Autodesk Inventor part; units mm, degrees
ref_plane "YZ Plane" through (0, 0, 0) normal (1, 0, 0) x (0, 1, 0)
ref_plane "XZ Plane" through (0, 0, 0) normal (0, 1, 0) x (-1, 0, 0)
ref_plane "XY Plane" through (0, 0, 0) normal (0, 0, 1) x (1, 0, 0)
sketch "スケッチ1" plane through (0, 0, 0) normal (1, 0, 0) x (0, 1, 0)
  line L0 (0, 0) -> (15, 0)
  line L1 (15, 0) -> (15, -150)
  line L2 (15, -150) -> (0, -150)
  line L3 (0, -150) -> (0, 0)
  line L4 (0, 0) -> (-40, 0)
  line L5 (-40, 0) -> (-40, -15)
  line L6 (-40, -15) -> (0, -15)
  line L7 (0, -15) -> (0, 0)
  line L8 (0, -150) -> (-40, -150)
  line L9 (-40, -150) -> (-40, -135)
  line L10 (-40, -135) -> (0, -135)
  line L11 (0, -135) -> (0, -150)
  dimension "d0" = 15
  dimension "d1" = 150
  dimension "d2" = 40
  dimension "d3" = 15
  dimension "d4" = 40
  dimension "d5" = 15
extrude "押し出し1" add sketch "スケッチ1" along normal blind 6
sketch "スケッチ2" plane through (6, 0, 0) normal (1, 0, 0) x (0, 0, -1)
  line L0 (150, 15) -> (0, 15)
  line L1 (0, 15) -> (0, -40)
  line L2 (75, 15) -> (75, -40) construction
  point P0 (0, 0)
  point P1 (7.5, 5)
  point P2 (7.5, -5)
  point P3 (7.5, -15)
  point P4 (25, 7.5)
  point P5 (35, 7.5)
  point P6 (45, 7.5)
  point P7 (142.5, 5)
  point P8 (142.5, -5)
  point P9 (142.5, -15)
  point P10 (125, 7.5)
  point P11 (115, 7.5)
  point P12 (105, 7.5)
  dimension "d8" = 10
  dimension "d9" = 7.5
  dimension "d10" = 10
  dimension "d11" = 10
  dimension "d12" = 7.5
  dimension "d13" = 25
  dimension "d14" = 10
  dimension "d15" = 10
hole "穴1" at (6, 5, -7.5) at (6, -5, -7.5) at (6, -15, -7.5) at (6, 7.5, -25) at (6, 7.5, -35) at (6, 7.5, -45) at (6, -15, -142.5) at (6, -5, -142.5) at (6, 5, -142.5) at (6, 7.5, -125) at (6, 7.5, -115) at (6, 7.5, -105) direction (-1, 0, 0) diameter 3.2 end through all
fillet "フィレット1" radius 2 8 edges at (3, 15, 0) (3, -40, -135) (3, 15, -150) (3, -40, -150) (3, 0, -15) (3, -40, -15) (3, -40, 0) (3, 0, -135)
properties part number "射出_受け身" material "アセタール樹脂、白"
Work out the finished part from the listing and answer in its coordinate system (mm). A direction names the side the tool comes from. Coordinates: 2 decimals unless noted, no trailing zeros. Write each loop counter-clockwise with the first axis right and the second up, starting at its lowest first coordinate (ties: lowest second). Pieces come first, ordered by that corner, then holes. Notation, with made-up numbers: (25.5, 56) - (32.5, 56) arc R25 ccw to (32.5, 86) - close; hole circle Ø2 at (-38.5, 40). An arc over 180 degrees is marked (long way). One line per question, with ' | ' between items.
1) For faces 5 (the face through (3, 15, -74)), 6 (the face through (3, -20, -135)), determine the directions among +Z, -Z, +X, -X, +Y, -Y from which every point of the face is accessible in a straight line to the end or side of a thin tool.
Checks:
face 5: +Z, -Z, +X, -X, +Y | face 6: +X, -X, -Y
2) Find section A-A, the plane y = -23. Determine the outline of the cut face in (x, z).
Checks:
outline: (0, -150) - (6, -150) - (6, -135) - (0, -135) - close; (0, -15) - (6, -15) - (6, 0) - (0, 0) - close
3) Consider probe 1 along Z at (x, y) = (3.3, -15); probe 2 along Y at (x, z) = (3.6, -142.5); probe 3 along Z at (x, y) = (4.1, 5). Determine where each line is inside the solid, lowest interval first. Write a range as [from, to].
Checks:
probe 1: [-150, -144.1], [-140.9, -135], [-15, -9.1], [-5.9, 0] | probe 2: [-40, -16.6], [-13.4, -6.6], [-3.4, 3.4], [6.6, 15] | probe 3: [-150, -144.1], [-140.9, -9.1], [-5.9, 0]
4) Find section D-D, the plane z = -35. Determine the outline of the cut face in (x, y).
Checks:
outline: (0, 0) - (6, 0) - (6, 5.9) - (0, 5.9) - close; (0, 9.1) - (6, 9.1) - (6, 15) - (0, 15) - close
5) Flat-ended cylindrical pins translate along their axes: P1, Ø4, axis at y = 7.5, z = -125, coming from the +X side; P2, Ø3, axis at x = 2.5, z = -54, coming from the -Y side. Find the tip coordinate at first contact, or state that the pin passes through.
Checks:
P1: x = 6 | P2: y = 0
6) Find section C-C, the plane y = -5. Determine the outline of the cut face in (x, z).
Checks:
outline: (0, -150) - (6, -150) - (6, -144.1) - (0, -144.1) - close; (0, -140.9) - (6, -140.9) - (6, -135) - (0, -135) - close; (0, -15) - (6, -15) - (6, -9.1) - (0, -9.1) - close; (0, -5.9) - (6, -5.9) - (6, 0) - (0, 0) - close
7) The mould has two halves that part along Y. Classify faces 1 (the face through (0, 5, -74)), 2 (the face through (2.958, -15.481, -144.026)), 3 (the face through (3, -40, -143)), 4 (the face through (2.96, 8.47, -33.73)): +Y half, -Y half, draft (parallel to the pull), parting line (faces both ways), or undercut.
Checks:
face 1: draft | face 2: undercut | face 3: -Y half | face 4: undercut
8) Find section B-B, the plane z = -7.5. Determine the outline of the cut face in (x, y), and give its area (3 significant figures).
Checks:
outline: (0, -40) - (6, -40) - (6, -16.6) - (0, -16.6) - close; (0, -13.4) - (6, -13.4) - (6, -6.6) - (0, -6.6) - close; (0, -3.4) - (6, -3.4) - (6, 3.4) - (0, 3.4) - close; (0, 6.6) - (6, 6.6) - (6, 15) - (0, 15) - close | area: 272 mm2
